The listing builds one solid part. Answer for the finished solid, in the listing's coordinates (mm). A direction names the side the tool comes from. Give positions to 0.01 mm unless a question says otherwise; leave off trailing zeros. Order: outer loops, then holes, each group sorted by start corner. A loop starts at its lowest first (then second) coordinate and runs counter-clockwise, first axis right, second up. Notation, with made-up numbers: (-11.5, 67) - (15.5, 67) arc R22 ccw to (15.5, 105) - close; hole circle Ø5 at (0, 27). An arc over 180 degrees is marked (long way). Write each question's results on one line, items separated by ' | '. Start each with the question number.
1. Which of the six approach directions +Z, -Z, +X, -X, +Y, -Y give full straight-line access (tool end or side, diameter ignored) to faces 1 (the face through (6.7, -2.1, 4.1)), 2 (the face through (0.983, -8.198, 4.056)), 3 (the face through (7.198, 4.045, 4.056))?
2. Section B-B (y = -11) is taken. Give the vertices of the cut face in (x, z), and give its area (3 significant figures).
3. Determine the mould class of faces 4 (the face through (8.198, 0.983, 4.056)), 5 (the face through (5.398, 4.512, 4.056)), 6 (the face through (-6.23, 3.26, 4.06)), 7 (the face through (0.623, -6.993, 4.056)) for opening direction X: released by +X, released by -X, zero draft, split by the parting line, or undercut.
4. Flat-ended cylindrical pins translate along their axes: pin 1 (1 mm diameter, centred on x = 4.5, z = 3.5, fed in from +Y); pin 2 (0.8 mm diameter, centred on y = 0, z = 4, fed in from +X); pin 3 (3.5 mm diameter, centred on y = 13.5, z = -5, fed in from +X); pin 4 (13 mm diameter, centred on x = -7, y = -3.5, fed in from +Z). Find the tip coordinate at first contact, or state that the pin passes through.
5. Section A-A (y = 0) is taken. Give the vertices of the cut face in (x, z), and give its area (3 significant figures).
6. Find the intervals of material crossed by L1, parallel to Y at x = 6.75, z = 6; L2, parallel to Y at x = -6, z = 6.75; L3, parallel to Y at x = 0, z = 3.5, in increasing order.
from build123d import *

# Parameters (mm, degrees)
PAD_DEPTH          = 7
SKETCH001_R        = 9
PAD001_DEPTH       = 8
POCKET_DEPTH       = 8
SKETCH003_R        = 2.6
POCKET001_DEPTH    = 16
POLARPATTERN_COUNT = 16
CHAMFER_SIZE       = 0.4


with BuildPart() as part:
    # Sketch → Pad (new body)
    with BuildSketch(Plane.XY):
        with BuildLine():
            ThreePointArc((0, -13), (11, -2), (0, 9))
            Line((0, 17), (0, 9))
            ThreePointArc((0, 17), (-15, 2), (0, -13))
        make_face()
    extrude(amount=-PAD_DEPTH)

    # Sketch001 (on Face4 of Pad) → Pad001 (join)
    with BuildSketch(Plane.XY):
        Circle(SKETCH001_R)
    extrude(amount=PAD001_DEPTH)

    # Sketch002 (on Face7 of Pad001) → Pocket (cut)
    with BuildSketch(Plane.XY.offset(8)):
        Polygon((1.25, 9), (0.75, 7.5), (0.5, 6.5), (-0.5, 6.5), (-0.75, 7.5), (-1.25, 9), align=None)
    pocket = extrude(amount=-POCKET_DEPTH, mode=Mode.SUBTRACT)

    # Sketch003 (on Face7 of Pad001) → Pocket001 (cut)
    with BuildSketch(Plane.XY.offset(8)):
        Circle(SKETCH003_R)
    extrude(amount=-POCKET001_DEPTH, mode=Mode.SUBTRACT)

    # PolarPattern: Pocket ×16 about axis
    polarpattern_axis = Axis((0, 0, 8), (0, 0, 1))
    for i in range(1, POLARPATTERN_COUNT):
        add(pocket.rotate(polarpattern_axis, i * 360 / POLARPATTERN_COUNT), mode=Mode.SUBTRACT)

    # Chamfer
    chamfer_edges = [part.edges().sort_by_distance(p)[0] for p in [
        (-2.6, 0, 8),
        (-2.6, 0, -7),
    ]]
    chamfer(chamfer_edges, length=CHAMFER_SIZE)


solid = part.part
Reported:
1) face 1: +Z | face 2: +Z, -Y | face 3: +Z, +X
2) outline: (-7.48, -7) - (6.32, -7) - (6.32, 0) - (-7.48, 0) - close | area: 96.7 mm²
3) face 4: released by +X | face 5: undercut | face 6: released by -X | face 7: undercut
4) pin 1: y = 7.77 | pin 2: x = 6.5 | pin 3: x = 0 | pin 4: z = 8
5) outline: (-14.87, -7) - (-3, -7) - (-2.6, -6.6) - (-2.6, 7.6) - (-3, 8) - (-6.5, 8) - (-6.5, 0) - (-14.87, 0) - close; (2.6, -6.6) - (3, -7) - (10.82, -7) - (10.82, 0) - (6.5, 0) - (6.5, 8) - (3, 8) - (2.6, 7.6) - close | area: 205 mm²
6) L1: -5.23 to -3.66, -2.11 to -0.56, 0.56 to 2.11, 3.66 to 5.23 | L2: -4.86 to -3.09, -2.5 to 2.5, 3.09 to 4.86 | L3: -6.5 to -2.6, 2.6 to 6.5
